Geometry check sheet. Reference: the model listing, model coordinates, mm. A direction names the side the tool comes from. Round coordinates to 2 decimals unless told otherwise and drop trailing zeros. Write each loop counter-clockwise with the first axis right and the second up, starting at its lowest first coordinate (ties: lowest second). Pieces come first, ordered by that corner, then holes. Notation, with made-up numbers: (40.5, 29) - (61.5, 29) arc R33 cw to (61.5, 62) - close; hole circle Ø1 at (51.5, -1). An arc over 180 degrees is marked (long way). Return JSON: item names as keys, results as strings.
```python
from build123d import *

# Parameters (mm, degrees)
BOSS_EXTRUDE1_DEPTH     = 1.375
CUT_EXTRUDE1_DEPTH      = 14.125518547
CUT_EXTRUDE1_DEPTH_BACK = 14.125518547
SKETCH2_R               = 0.75


with BuildPart() as part:
    # Sketch1 → Boss-Extrude1 (new, symmetric)
    with BuildSketch(Plane.XY):
        with BuildLine():
            Line((-8.65, 0), (-6.482615316, 0))
            ThreePointArc((-6.482615316, 0), (-5.637378793, -0.187384426), (-4.95052643, -0.714424781))
            Line((-4.95052643, -0.714424781), (-3.602119315, -2.321393805))
            ThreePointArc((-3.602119315, -2.321393805), (-3.430406224, -2.453153894), (-3.219097093, -2.5))
            Line((-3.219097093, -2.5), (3.219097093, -2.5))
            ThreePointArc((3.219097093, -2.5), (3.430406224, -2.453153894), (3.602119315, -2.321393805))
            Line((3.602119315, -2.321393805), (4.95052643, -0.714424781))
            ThreePointArc((4.95052643, -0.714424781), (5.637378793, -0.187384426), (6.482615316, 0))
            Line((6.482615316, 0), (8.65, 0))
            ThreePointArc((8.65, 0), (9.074264069, -0.175735931), (9.25, -0.6))
            Line((9.25, -0.6), (9.25, -0.9))
            ThreePointArc((9.25, -0.9), (9.074264069, -1.324264069), (8.65, -1.5))
            Line((8.65, -1.5), (6.35, -1.5))
            ThreePointArc((6.35, -1.5), (6.137867966, -1.587867966), (6.05, -1.8))
            Line((6.05, -1.8), (6.05, -2))
            ThreePointArc((6.05, -2), (4.337132574, -6.706064576), (0, -9.210109235))
            ThreePointArc((0, -9.210109235), (-4.337132574, -6.706064576), (-6.05, -2))
            Line((-6.05, -2), (-6.05, -1.8))
            ThreePointArc((-6.05, -1.8), (-6.137867966, -1.587867966), (-6.35, -1.5))
            Line((-6.35, -1.5), (-8.65, -1.5))
            ThreePointArc((-8.65, -1.5), (-9.074264069, -1.324264069), (-9.25, -0.9))
            Line((-9.25, -0.9), (-9.25, -0.6))
            ThreePointArc((-9.25, -0.6), (-9.074264069, -0.175735931), (-8.65, 0))
        make_face()
        with BuildLine():
            Line((2.989643947, -4.25), (-2.989643947, -4.25))
            ThreePointArc((-2.989643947, -4.25), (-3.428714462, -4.510799074), (-3.409748242, -5.021131667))
            ThreePointArc((-3.409748242, -5.021131667), (-1.938287409, -6.553911081), (0, -7.424342947))
            ThreePointArc((0, -7.424342947), (1.938287409, -6.553911081), (3.409748242, -5.021131667))
            ThreePointArc((3.409748242, -5.021131667), (3.428714462, -4.510799074), (2.989643947, -4.25))
        make_face(mode=Mode.SUBTRACT)
    extrude(amount=BOSS_EXTRUDE1_DEPTH, both=True)

    # Sketch2 → Cut-Extrude1 (cut, two sides: drawn at the far end of the back side and taken through both)
    with BuildSketch(Plane(origin=(0, 0, 0), x_dir=(1, 0, 0), z_dir=(0, 1, 0)).offset(-CUT_EXTRUDE1_DEPTH_BACK)):
        with Locations(Location((0, 0, 0), (0, 0, 270))):
            Circle(SKETCH2_R)
        with Locations(Location((-7.5, 0, 0), (0, 0, 180))):
            Circle(SKETCH2_R)
        with Locations((7.5, 0)):
            Circle(SKETCH2_R)
    extrude(amount=CUT_EXTRUDE1_DEPTH + CUT_EXTRUDE1_DEPTH_BACK, mode=Mode.SUBTRACT)


solid = part.part
```
(1) Section check A-A, the plane x = -7.5. Enter the section's corners in (y, z) (3 decimals).
Response values:
{"outline": "(-1.5, -1.375) - (0, -1.375) - (0, -0.75) - (-1.5, -0.75) - close; (-1.5, 0.75) - (0, 0.75) - (0, 1.375) - (-1.5, 1.375) - close"}
(2) Section check D-D, the plane y = -6. Enter the section's corners in (x, z) (3 decimals).
Response values:
{"outline": "(-4.861, -1.375) - (-2.607, -1.375) - (-2.607, 1.375) - (-4.861, 1.375) - close; (2.607, -1.375) - (4.861, -1.375) - (4.861, 1.375) - (2.607, 1.375) - close"}
(3) Section check B-B, the plane z = 1.15. Enter the section's corners in (x, y).
Response values:
{"outline": "(-9.25, -0.9) arc R0.6 ccw to (-8.65, -1.5) - (-6.35, -1.5) arc R0.3 cw to (-6.05, -1.8) - (-6.05, -2) arc R7.32 ccw to (0, -9.21) arc R7.32 ccw to (6.05, -2) - (6.05, -1.8) arc R0.3 cw to (6.35, -1.5) - (8.65, -1.5) arc R0.6 ccw to (9.25, -0.9) - (9.25, -0.6) arc R0.6 ccw to (8.65, 0) - (6.48, 0) arc R2 ccw to (4.95, -0.71) - (3.6, -2.32) arc R0.5 cw to (3.22, -2.5) - (-3.22, -2.5) arc R0.5 cw to (-3.6, -2.32) - (-4.95, -0.71) arc R2 ccw to (-6.48, 0) - (-8.65, 0) arc R0.6 ccw to (-9.25, -0.6) - close; hole (-3.41, -5.02) arc R5.57 ccw to (0, -7.42) arc R5.57 ccw to (3.41, -5.02) arc R0.5 ccw to (2.99, -4.25) - (-2.99, -4.25) arc R0.5 ccw to start"}
(4) Section check C-C, the plane y = -4. Enter the section's corners in (x, z) (3 decimals), plus the area to 3 significant figures.
Response values:
{"outline": "(-5.772, -1.375) - (5.772, -1.375) - (5.772, 1.375) - (-5.772, 1.375) - close; hole circle Ø1.5 at (0, 0)", "area": "30.0 mm^2"}
(5) Access from +Z, -Z, +X, -X, +Y, -Y to the whole of each face (thin tool, end or side, straight path). Record for faces 1 (the face through (-8, -1.5, -1)), 2 (the face through (1.914, -6.571, 0.019)), 3 (the face through (5.63, -0.19, 0.02)).
Response values:
{"face 1": "+Z, -Z, -X, -Y", "face 2": "+Z, -Z", "face 3": "+Z, -Z, +Y"}
(6) Release check for a two-part mould opening along Z. For faces 4 (the face through (0, -4, -1.375)), 5 (the face through (7, -1.5, -1)), 6 (the face through (0.225, -3.387, 0.715)) record: pulls with the +Z half, pulls with the -Z half, needs draft (parallel to the pull), parting line crosses it, or undercut.
Response values:
{"face 4": "pulls with the -Z half", "face 5": "needs draft", "face 6": "undercut"}
(7) Gauge pin test, flat ends, axial feed: pin 1 (1.5 mm diameter, centred on x = 2.5, y = -2, fed in from -Z) (3 decimals); pin 2 (1.4 mm diameter, centred on x = 0, z = -0.5, fed in from +Y). Record the tip position at first contact, or that the pin passes through.
Response values:
{"pin 1": "stops at z = -1.375", "pin 2": "stops at y = -2.5"}
(8) Material ranges on line 1 along Z through (x, y) = (0, -8.35) (3 decimals); line 2 along Y through (x, z) = (7.75, 0.75); line 3 along Y through (x, z) = (-1.75, 0.1), recorded low to high. Write a range as [from, to].
Response values:
{"line 1": "z = [-1.375, -0.75], [0.75, 1.375]", "line 2": "y = [-1.5, 0]", "line 3": "y = [-8.67, -6.68], [-4.25, -2.5]"}
